The listing builds one solid part. Answer for the finished solid, in the listing's coordinates (mm). Face numbers are marked on the shaded views. A direction names the side the tool comes from. Coordinates: 2 decimals unless noted, no trailing zeros. Order: outer loops, then holes, each group sorted by start corner. A loop starts at its lowest first (then second) coordinate and runs counter-clockwise, first axis right, second up.
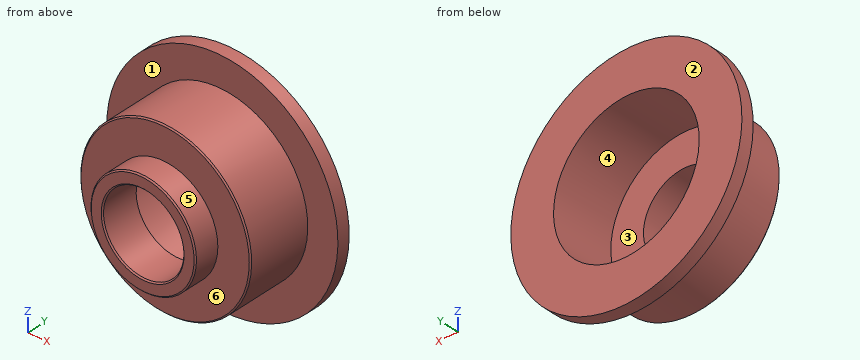
Autodesk Inventor part; units mm, degrees
ref_plane "YZ Plane" through (0, 0, 0) normal (1, 0, 0) x (0, 1, 0)
ref_plane "XZ Plane" through (0, 0, 0) normal (0, 1, 0) x (-1, 0, 0)
ref_plane "XY Plane" through (0, 0, 0) normal (0, 0, 1) x (1, 0, 0)
sketch "Skizze1" plane through (0, 0, 0) normal (1, 0, 0) x (0, 1, 0)
  line L0 (0, -16) -> (-5, -16)
  line L1 (-5, -16) -> (-5, -34)
  line L2 (-5, -34) -> (0, -34)
  line L3 (0, -34) -> (0, -16)
  line L4 (-11.0954, 0) -> (31.5723, 0)
  line L5 (0, -55.2) -> (0, 9.2)
  line L6 (0, -34) -> (25.477, -34)
  line L7 (25.477, -34) -> (25.477, -29)
  line L8 (25.477, -29) -> (0, -29)
  line L9 (0, -29) -> (0, -34)
  line L10 (25.477, -34) -> (20.477, -34)
  line L11 (20.477, -34) -> (20.477, -46)
  line L12 (20.477, -46) -> (25.477, -46)
  line L13 (25.477, -46) -> (25.477, -34)
  point P0 (0, 0)
  point P1 (0, -29)
  dimension "d0" = 16
  dimension "d1" = 34
  dimension "d2" = 5
  dimension "d3" = 5
  dimension "d4" = 5
  dimension "d5" = 46
revolve "Umdrehung1" add sketch "Skizze1" angle 360 about axis through (0, -10, 0) along (0, 1, 0)
chamfer "Fase1" distance 0.5 angle 45 1 edges at (0, -5, 34)
sketch "Skizze2" plane through (0, -5, 0) normal (0, -1, 0) x (1, 0, 0)
  circle A0 centre (0, 0) radius 16
  circle A1 centre (0, 0) radius 21
  circle A2 centre (0, 0) radius 16
  dimension "d10" = 5
  dimension "d11" = 0
extrude "Extrusion1" add sketch "Skizze2" along normal blind 10
chamfer "Fase2" distance 0.5 angle 45 2 edges at (-21, -15, 0) (-16, -15, 0)
equation "\"d3\" = d2"
equation "\"d4\" = d2"
properties part number "Topf"
(1) Each of these flat-tipped pins is pushed along its axis until it touches: pin 1 Ø8 at (x, z) = (28, -32.5) entering from -Y; pin 2 Ø6 at (x, y) = (-0.5, -7) entering from -Z; pin 3 Ø4 at (y, z) = (0, 22) entering from +X. Where does it stop, or does it pass through?
(2) Consider line 1 (X direction, y = -4, z = 0); line 2 (Z direction, x = 0, y = 9.75). Determine where each line is inside the solid, lowest interval first.
(3) Find section B-B (z = 0). Write down the section's boundary in (x, y), and give its area (3 significant figures).
(4) Find section C-C (y = 5.5). Write down the section's boundary in (x, z).
(5) The mould has two halves that part along Z. Classify the marked faces 4, 5 and 6: released by +Z, released by -Z, zero draft, split by the parting line, or undercut.
(6) Find section A-A (x = 0). Write down the section's boundary in (y, z).
(7) Find section D-D (x = 37). Write down the section's boundary in (y, z), and give its area (3 significant figures).
(8) For the marked faces 1, 2 and 3, determine the directions among +Z, -Z, +X, -X, +Y, -Y from which every point of the face is accessible in a straight line to the end or side of a thin tool.
Findings below:
1. pin 1: stops at y = 20.48
1. pin 2: stops at z = -34
1. pin 3: stops at x = 27.5
2. line 1: x = -34 to -16, 16 to 34
2. line 2: z = -34 to -29, 29 to 34
3. outline: (-46, 20.48) - (-34, 20.48) - (-34, -4.5) - (-33.5, -5) - (-21, -5) - (-21, -14.5) - (-20.5, -15) - (-16.5, -15) - (-16, -14.5) - (-16, 0) - (-29, 0) - (-29, 25.48) - (-46, 25.48) - close; (16, -14.5) - (16.5, -15) - (20.5, -15) - (21, -14.5) - (21, -5) - (33.5, -5) - (34, -4.5) - (34, 20.48) - (46, 20.48) - (46, 25.48) - (29, 25.48) - (29, 0) - (16, 0) - close
3. area: 654 mm2
4. outline: circle Ø68 at (0, 0); hole circle Ø58 at (0, 0)
5. face 4: undercut
5. face 5: split by the parting line
5. face 6: zero draft
6. outline: (-15, -20.5) - (-14.5, -21) - (-5, -21) - (-5, -33.5) - (-4.5, -34) - (20.48, -34) - (20.48, -46) - (25.48, -46) - (25.48, -29) - (0, -29) - (0, -16) - (-14.5, -16) - (-15, -16.5) - close; (-15, 16.5) - (-14.5, 16) - (0, 16) - (0, 29) - (25.48, 29) - (25.48, 46) - (20.48, 46) - (20.48, 34) - (-4.5, 34) - (-5, 33.5) - (-5, 21) - (-14.5, 21) - (-15, 20.5) - close
7. outline: (20.48, -27.33) - (25.48, -27.33) - (25.48, 27.33) - (20.48, 27.33) - close
7. area: 273 mm2
8. face 1: -Y
8. face 2: +Z, -Z, +X, -X, +Y
8. face 3: +Y
